Here's how the part is built. I have some questions about the finished solid (model axes, mm). A direction names the side the tool comes from. Give positions to 0.01 mm unless a question says otherwise; leave off trailing zeros. Write each loop counter-clockwise with the first axis right and the second up, starting at its lowest first coordinate (ties: lowest second). Pieces come first, ordered by that corner, then holes. Notation, with made-up numbers: (-28.75, -23) -> (10.25, -23) arc R20 ccw to (10.25, -4) -> close; hole circle Ø3 at (85.25, -8). An arc over 180 degrees is marked (long way). Return JSON: item names as keys, results as strings.
from build123d import *

# Parameters (mm, degrees)
SKETCH1_W           = 200
SKETCH1_H           = 150
BOSS_EXTRUDE1_DEPTH = 10
SKETCH2_R           = 10
CUT_EXTRUDE1_DEPTH  = 10
SKETCH4_W           = 150
SKETCH4_H           = 10
BOSS_EXTRUDE2_DEPTH = 20
SKETCH3_W           = 20
SKETCH3_H           = 60
BOSS_EXTRUDE3_DEPTH = 25
SKETCH5_W           = 20
SKETCH5_H           = 60
SKETCH5_W_2         = 40
SKETCH5_H_2         = 200
BOSS_EXTRUDE4_DEPTH = 25
SKETCH7_R           = 5
CUT_EXTRUDE3_DEPTH  = 251
SKETCH9_R           = 10
CUT_EXTRUDE4_DEPTH  = 241


with BuildPart() as part:
    # Sketch1 → Boss-Extrude1 (new body)
    with BuildSketch(Plane(origin=(0, 0, 0), x_dir=(1, 0, 0), z_dir=(0, 1, 0))):
        Rectangle(SKETCH1_W, SKETCH1_H)
    extrude(amount=BOSS_EXTRUDE1_DEPTH)

    # Sketch2 → Cut-Extrude1 (cut)
    with BuildSketch(Plane(origin=(0, 10, 0), x_dir=(1, 0, 0), z_dir=(0, 1, 0))):
        with Locations(Location((50, 0, 0), (0, 0, 270))):
            Circle(SKETCH2_R)
    extrude(amount=-CUT_EXTRUDE1_DEPTH, mode=Mode.SUBTRACT)

    # Sketch4 → Boss-Extrude2 (add)
    with BuildSketch(Plane.ZY.offset(100)):
        with Locations((0, 5)):
            Rectangle(SKETCH4_W, SKETCH4_H)
    extrude(amount=BOSS_EXTRUDE2_DEPTH)

    # Sketch3 → Boss-Extrude3 (add)
    with BuildSketch(Plane.XY.offset(75)):
        with Locations((90, 30)):
            Rectangle(SKETCH3_W, SKETCH3_H)
        Polygon((-100, 200), (-120, 200), (-120, 0), (-100, 0), (-80, 0), (-80, 200), align=None)
    extrude(amount=BOSS_EXTRUDE3_DEPTH)

    # Sketch5 → Boss-Extrude4 (add)
    with BuildSketch(Plane(origin=(0, 0, -75), x_dir=(-1, 0, 0), z_dir=(0, 0, -1))):
        with Locations((-90, 30)):
            Rectangle(SKETCH5_W, SKETCH5_H)
        with Locations((100, 100)):
            Rectangle(SKETCH5_W_2, SKETCH5_H_2)
    extrude(amount=BOSS_EXTRUDE4_DEPTH)

    # Sketch7 → Cut-Extrude3 (cut)
    with BuildSketch(Plane(origin=(0, 0, -100), x_dir=(-1, 0, 0), z_dir=(0, 0, -1))):
        with Locations((-90, 40)):
            Circle(SKETCH7_R)
    extrude(amount=-CUT_EXTRUDE3_DEPTH, mode=Mode.SUBTRACT)

    # Sketch9 → Cut-Extrude4 (cut)
    with BuildSketch(Plane.XY.offset(100)):
        with Locations((-100, 160)):
            Circle(SKETCH9_R)
        with Locations((-100, 135)):
            Circle(SKETCH9_R)
        with Locations((-100, 110)):
            Circle(SKETCH9_R)
        with Locations((-100, 85)):
            Circle(SKETCH9_R)
        with Locations((-100, 35)):
            Circle(SKETCH9_R)
        with Locations((-100, 60)):
            Circle(SKETCH9_R)
    extrude(amount=-CUT_EXTRUDE4_DEPTH, mode=Mode.SUBTRACT)


solid = part.part
1. Suppose I cut it at A-A, the plane y = 85. List the corners of the cut face in (x, z) for me, and give its area (3 significant figures).
Taken from the geometry:
{"outline": "(-120, -100) -> (-110, -100) -> (-110, -75) -> (-120, -75) -> close; (-120, 75) -> (-110, 75) -> (-110, 100) -> (-120, 100) -> close; (-90, -100) -> (-80, -100) -> (-80, -75) -> (-90, -75) -> close; (-90, 75) -> (-80, 75) -> (-80, 100) -> (-90, 100) -> close", "area": "1,000 mm²"}
2. Which directions (+Z, -Z, +X, -X, +Y, -Y) give clear straight access to the entire face, cutting with the end or side of a thin tool? Please do faces 4 (the face through (1, 5, -75)), 5 (the face through (-107.37, 141.76, 87.68)), 6 (the face through (-8, 10, -1)).
Taken from the geometry:
{"face 4": "-Z, +Y, -Y", "face 5": "+Z, -Z", "face 6": "+X, -X, +Y"}
3. For pin 1 Ø12 at (x, z) = (-91, -61.5) entering from +Y; pin 2 Ø12 at (x, y) = (-98.5, 63) entering from +Z; pin 3 Ø11 at (x, y) = (29, 5.5) entering from -Z; pin 4 Ø16 at (x, z) = (92, 87.5) entering from +Y, each with a flat end and sliding along its axis, tell me the tip position at first contact or that it passes through.
Taken from the geometry:
{"pin 1": "stops at y = 10", "pin 2": "passes through", "pin 3": "stops at z = -75", "pin 4": "stops at y = 60"}
4. Suppose I cut it at B-B, the plane z = 0. List the corners of the cut face in (x, y) for me, and give its area (3 significant figures).
Taken from the geometry:
{"outline": "(-120, 0) -> (40, 0) -> (40, 10) -> (-120, 10) -> close; (60, 0) -> (100, 0) -> (100, 10) -> (60, 10) -> close", "area": "2,000 mm²"}
5. Suppose I cut it at C-C, the plane x = -100. Count the separate pieces of the cut face and the enclosed holes in it, and give its area (3 significant figures).
Taken from the geometry:
{"separate pieces": "13", "enclosed holes": "0", "area": "5,500 mm²"}
6. If we mould it in two halves opening along X, with no side actions, what happens to faces 1 (the face through (-120, 86, -82)), 2 (the face through (92, 35, 75)), 3 (the face through (-108, 29, -87))? For each: released by +X, released by -X, zero draft, split by the parting line, or undercut.
Taken from the geometry:
{"face 1": "released by -X", "face 2": "zero draft", "face 3": "undercut"}
7. If I drill on line 1 (Y direction, x = 90, z = -93); line 2 (Z direction, x = -80.5, y = 52); line 3 (Y direction, x = 60.5, z = 15.5), over which ranges is the centre line in solid material (lowest first)? Write a range as [from, to].
Taken from the geometry:
{"line 1": "y = [0, 35], [45, 60]", "line 2": "z = [-100, -75], [75, 100]", "line 3": "y = [0, 10]"}
